Geometry check sheet. Reference: drawing and pictorial views, mm from the part's lowest x, y, z. Round coordinates to 2 decimals unless told otherwise and drop trailing zeros. Write each loop counter-clockwise with the first axis right and the second up, starting at its lowest first coordinate (ties: lowest second). Pieces come first, ordered by that corner, then holes. Notation, with made-up numbers: M -24.5,8 L 32.5,8 A17 cw 32.5,30 Z; hole C 16,35.25 d3. An arc over 180 degrees is marked long. Answer in a Markdown table with one row per item. Add a question column.
1. Sectioned sample at B-B on z = 20.5. Record the cut outline in (x, y), plus the area to 3 significant figures.
2. Go/stop test with a flat-tipped pin: pin 1 Ø2.5 at (x, y) = (9.5, 34.5) entering from -Z. Record where the tip stops, or that it passes through.
3. Sectioned sample at D-D on z = 2.25. Count the separate pieces of the cut face and the enclosed holes in it, plus the area to 3 significant figures.
4. Sectioned sample at C-C on y = 31.5. Record the cut outline in (x, z).
5. Material ranges on probe 1 along Y at (x, z) = (9.6, 2); probe 2 along Z at (x, y) = (50, 13); probe 3 along X at (y, z) = (36, 18.5), recorded low to high.
6. Sectioned sample at A-A on x = 35. Record the cut outline in (y, z), plus the area to 3 significant figures.
7. Draft check along X on the marked faces 1, 2, 3 and 4. Enter one of: pulls with the +X half, pulls with the -X half, needs draft (parallel to the pull), parting line crosses it, or undercut.
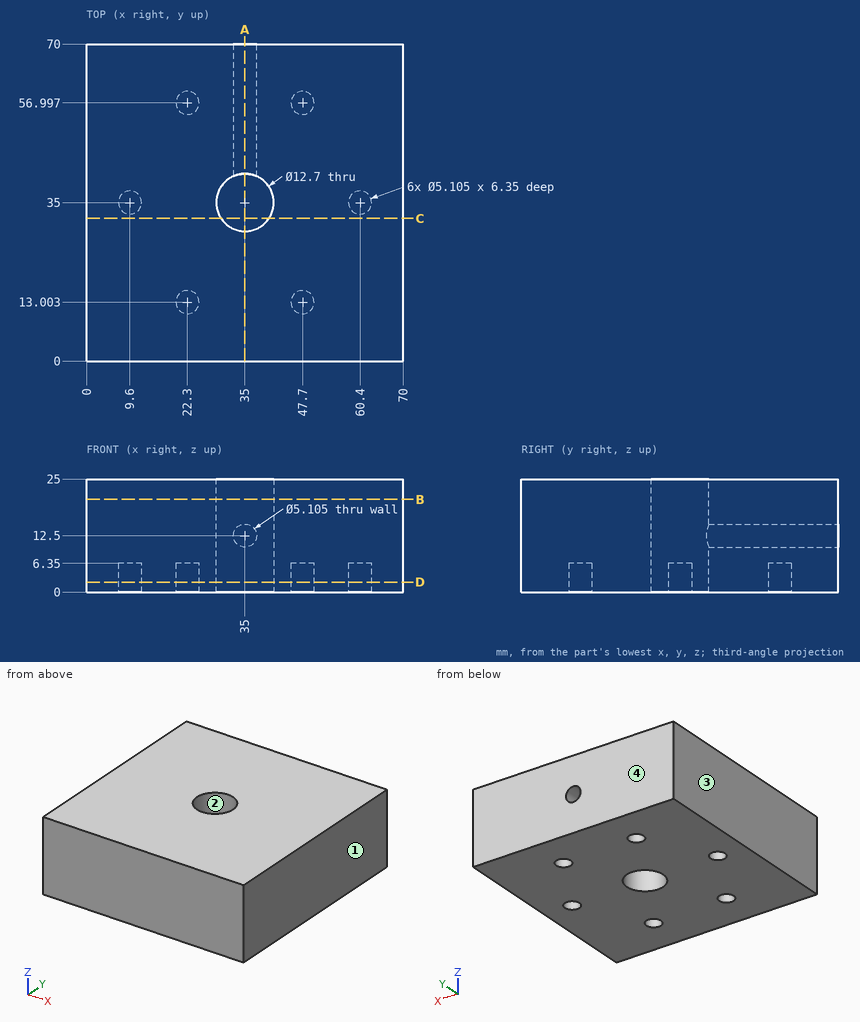
Geometry check:
| question | item | result |
|---|---|---|
| 1 | outline | M 0,0 L 70,0 L 70,70 L 0,70 Z; hole C 35,35 d12.7 |
| 1 | area | 4,770 mm2 |
| 2 | pin 1 | stops at z = 6.35 |
| 3 | separate pieces | 1 |
| 3 | enclosed holes | 7 |
| 3 | area | 4,650 mm2 |
| 4 | outline | M 0,0 L 29.7,0 L 29.7,25 L 0,25 Z; M 40.3,0 L 70,0 L 70,25 L 40.3,25 Z |
| 5 | probe 1 | y = 0 to 32.45, 37.55 to 70 |
| 5 | probe 2 | z = 6.35 to 25 |
| 5 | probe 3 | x = 0 to 28.73, 41.27 to 70 |
| 6 | outline | M 0,0 L 28.65,0 L 28.65,25 L 0,25 Z; M 41.35,0 L 70,0 L 70,9.95 L 41.35,9.95 Z; M 41.35,15.05 L 70,15.05 L 70,25 L 41.35,25 Z |
| 6 | area | 1,290 mm2 |
| 7 | face 1 | pulls with the +X half |
| 7 | face 2 | undercut |
| 7 | face 3 | pulls with the -X half |
| 7 | face 4 | needs draft |
